Geometry check sheet. Reference: the model listing, model coordinates, mm. A direction names the side the tool comes from. Round coordinates to 2 decimals unless told otherwise and drop trailing zeros. Return JSON: item names as keys, results as strings. Group by question number.
Q1. Sectioned sample at A-A, the plane z = 7.25. Give the number of separate pieces and of enclosed holes in the cut face, then the cut area to 3 significant figures.
Q2. Gauge pin test, flat ends, axial feed: pin 1 Ø0.5 at (x, z) = (3.5, 7) entering from -Y; pin 2 Ø1 at (y, z) = (0, 7.5) entering from -X; pin 3 Ø0.8 at (y, z) = (-0.5, 8) entering from +X. Record the tip position at first contact, or that the pin passes through.
Q3. Material ranges on line 1 along X through (y, z) = (0.35, 7.5); line 2 along Z through (x, y) = (2.5, -0.25); line 3 along Z through (x, y) = (2.45, 0.8), recorded low to high.
Q4. Tool access check on faces 4 (the flat face through (2.35, -0.6, 8)), 5 (the flat face through (3, -0.15, 8)). Record the directions out of +Z, -Z, +X, -X, +Y, -Y that give a thin tool (end or side, any length) a straight path to the whole face; none if there is none.
Q5. Draft check along Y on faces 1 (the flat face through (2, 0.15, 8)), 2 (the flat face through (2.65, -0.7, 8)), 3 (the cylindrical face through (3.095, 0.456, -0.789)). Enter one of: pulls with the +Y half, pulls with the -Y half, needs draft (parallel to the pull), parting line crosses it, or undercut.
```python
from build123d import *

# Parameters (mm, degrees)
EXTRUDE005_DEPTH = 4.5
SKETCH003_R      = 1
SKETCH004_R      = 1
SKETCH005_R      = 1.2
FILLET006_R      = 0.5
SKETCH007_R      = 0.75
EXTRUDE006_DEPTH = 2
FILLET013_R      = 0.4


with BuildPart() as extrude005:
    # Sketch006 → Extrude005 (new body)
    with BuildSketch(Plane.XY.offset(10.2)):
        Polygon((-2.65, 2.1), (-2.35, 2.1), (-2.35, 0.15), (-0.910869, 0.15), (-0.910869, -0.15), (-2.35, -0.15), (-2.35, -2.1), (-2.65, -2.1), (-2.65, -0.15), (-4.365716, -0.15), (-4.365716, 0.15), (-2.65, 0.15), align=None)
    extrude(amount=-EXTRUDE005_DEPTH)


with BuildPart() as cut002:
    # Sketch003 → Loft section 0
    with BuildSketch(Plane(origin=(0, 0, 0), x_dir=(1, 0, 0), z_dir=(0, 0, -1))):
        with Locations((-2.5, 0)):
            Circle(SKETCH003_R)
    # Sketch004 → Loft section 1
    with BuildSketch(Plane(origin=(0, 0, 6), x_dir=(1, 0, 0), z_dir=(0, 0, -1))):
        with Locations((-2.5, 0)):
            Circle(SKETCH004_R)
    # Sketch005 → Loft section 2
    with BuildSketch(Plane(origin=(0, 0, 10.2), x_dir=(1, 0, 0), z_dir=(0, 0, -1))):
        with Locations((-2.5, 0)):
            Circle(SKETCH005_R)
    loft()

    # Fillet006
    fillet006_edges = [cut002.edges().sort_by_distance(p)[0] for p in [
        (-3.7, 0, 10.2),
    ]]
    fillet(fillet006_edges, radius=FILLET006_R)

    # Cut002: cut Extrude005
    add(extrude005.part, mode=Mode.SUBTRACT)


with BuildPart() as pin003:
    # Sketch007 → Extrude006 (new body)
    with BuildSketch(Plane(origin=(0, 0, 0), x_dir=(1, 0, 0), z_dir=(0, 0, -1))):
        with Locations((-2.5, 0)):
            Circle(SKETCH007_R)
    extrude(amount=EXTRUDE006_DEPTH)

    # Fusion001: union Cut002
    add(cut002.part)

    # Fillet013
    fillet013_edges = [pin003.edges().sort_by_distance(p)[0] for p in [
        (-3.25, 0, -2),
    ]]
    fillet(fillet013_edges, radius=FILLET013_R)


with BuildPart() as part_mirroring:
    # Part__Mirroring: instance of pin003
    add(pin003.part.mirror(Plane(origin=(0, 0, 0), x_dir=(0, -1, 0), z_dir=(1, 0, 0))))


solid = part_mirroring.part
```
Reply:
{
 "1": {"separate pieces": "4", "enclosed holes": "0", "area": "2.26 mm^2"},
 "2": {"pin 1": "y = -0.71", "pin 2": "x = 1.44", "pin 3": "x = 3.57"},
 "3": {"line 1": "1.51 to 2.35, 2.65 to 3.49", "line 2": "-2 to 5.7", "line 3": "0 to 5.7"},
 "4": {"face 4": "+Z, +Y, -Y", "face 5": "+Z, +X, -X"},
 "5": {"face 1": "undercut", "face 2": "needs draft", "face 3": "parting line crosses it"}
}
